from build123d import *

# Parameters (mm, degrees)
BOSS_EXTRUDE1_DEPTH = 279.4
SKETCH2_W           = 241.3
SKETCH2_H           = 124.206
SKETCH2_H_2         = 28.194
CUT_EXTRUDE3_DEPTH  = 80.368181
FILLET1_R           = 1.5875
SKETCH4_W           = 241.3
SKETCH4_H           = 84.002363795
CUT_EXTRUDE5_DEPTH  = 7.62


with BuildPart() as part:
    # Sketch1 → Boss-Extrude1 (new body)
    with BuildSketch(Plane(origin=(0, 0, 0), x_dir=(0, 0, -1), z_dir=(1, 0, 0))):
        with BuildLine():
            Line((0, 0), (101.6, 0))
            Line((101.6, 0), (152.4, 87.988181024))
            Line((152.4, 87.988181024), (124.206, 87.988181024))
            ThreePointArc((124.206, 87.988181024), (89.315487923, 46.885255226), (43.091610276, 74.636858378))
            Line((43.091610276, 74.636858378), (0, 0))
        make_face()
        with BuildLine():
            Line((139.201772846, 80.368181024), (131.23325971, 80.368181024))
            ThreePointArc((131.23325971, 80.368181024), (94.185048049, 40.105513671), (42.791899046, 58.8777433))
            Line((42.791899046, 58.8777433), (13.198227154, 7.62))
            Line((13.198227154, 7.62), (97.200590949, 7.62))
            Line((97.200590949, 7.62), (139.201772846, 80.368181024))
        make_face(mode=Mode.SUBTRACT)
    extrude(amount=BOSS_EXTRUDE1_DEPTH)

    # Sketch2 → Cut-Extrude3 (cut)
    with BuildSketch(Plane(origin=(0, 87.988181024, 0), x_dir=(1, 0, 0), z_dir=(0, 1, 0))):
        with Locations((139.7, 62.103)):
            Rectangle(SKETCH2_W, SKETCH2_H)
        with Locations((139.7, 138.303)):
            Rectangle(SKETCH2_W, SKETCH2_H_2)
    extrude(amount=-CUT_EXTRUDE3_DEPTH, mode=Mode.SUBTRACT)

    # Fillet1
    fillet1_edges = [part.edges().sort_by_distance(p)[0] for p in [
        (279.4, 46.885255226, -89.315487923),
        (9.525, 74.636858378, -43.091610276),
        (9.525, 87.988181024, -124.206),
        (19.05, 46.885255226, -89.315487923),
        (260.35, 46.885255226, -89.315487923),
        (0, 46.885255226, -89.315487923),
        (269.875, 74.636858378, -43.091610276),
        (269.875, 87.988181024, -124.206),
    ]]
    fillet(fillet1_edges, radius=FILLET1_R)

    # Sketch4 → Cut-Extrude5 (cut)
    with BuildSketch(Plane(origin=(0, 7.62, 0), x_dir=(1, 0, 0), z_dir=(0, 1, 0))):
        with Locations((139.7, 55.199409051)):
            Rectangle(SKETCH4_W, SKETCH4_H)
    extrude(amount=-CUT_EXTRUDE5_DEPTH, mode=Mode.SUBTRACT)


solid = part.part
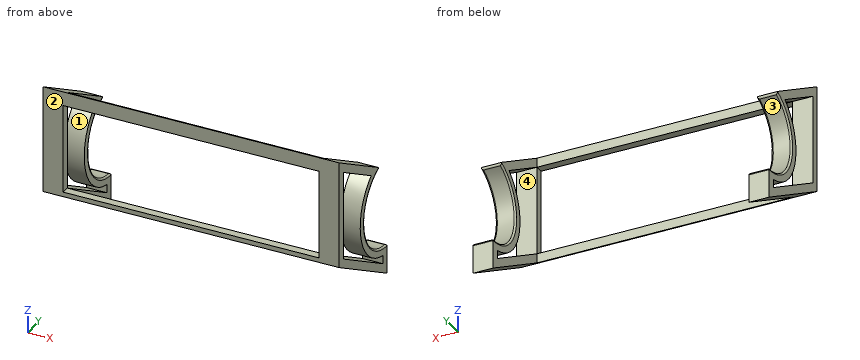
Design review of the part built by this model. Coordinates are the model's own, in mm. Face numbers are marked on the shaded views. A direction names the side the tool comes from. Coordinates: 2 decimals unless noted, no trailing zeros. Loops run counter-clockwise (first coordinate to the right, second up) from the corner with the lowest first, then second, coordinate; pieces in that order, holes last. Notation, with made-up numbers: (52, 33) -> (72, 33) arc R21 cw to (72, 56) -> close; hole circle Ø11 at (-11.5, 17.5). An arc over 180 degrees is marked (long way). Use a Markdown table: item, result. Add a question column.
Item 1: Clearance check with flat-ended pins moving along their axes: P1, Ø7, axis at x = 100.5, z = -100, coming from the +Y side; P2, Ø21, axis at x = 9, z = -44, coming from the +Y side; P3, Ø6, axis at x = 160, y = 4.5, coming from the +Z side. State where each tip first meets the part, or that it passes through.
Item 2: We need section C-C, the plane z = -34. Write out the cut boundary in (x, y), and give its area (3 significant figures).
Item 3: We need section D-D, the plane y = 20.5. Write out the cut boundary in (x, z).
Item 4: We need section B-B, the plane y = 42. Write out the cut boundary in (x, z), and give its area (3 significant figures).
Item 5: We need section A-A, the plane x = 34. Write out the cut boundary in (y, z), and give its area (3 significant figures).
Item 6: Machinability: for the marked faces 3 and 4, which of the approach directions +Z, -Z, +X, -X, +Y, -Y give a long, thin tool a straight path to every point of the face, cutting with its end or side? Answer none if there is none.
Item 7: The part is to be moulded in two halves that separate along Z. For the marked faces 1 and 2, say which applies: +Z half, -Z half, draft (parallel to the pull), parting line (faces both ways), or undercut.
Item 8: Wall thickness on L1, parallel to X at y = 4, z = -68; L2, parallel to Y at x = 123, z = -99.5; L3, parallel to Z at x = 76, y = 6: over which ranges is each line inside the solid? List them lowest first. Write a range as from..to.
Numbers:
| question | item | result |
|---|---|---|
| 1 | P1 | stops at y = 7.62 |
| 1 | P2 | stops at y = 72.55 |
| 1 | P3 | stops at z = -0.87 |
| 2 | outline | (0, 0) -> (19.05, 0) -> (19.05, 7.62) -> (0, 7.62) -> close; (0, 43.65) -> (19.05, 43.65) -> (19.05, 58.89) -> (0, 58.89) -> close; (260.35, 0) -> (279.4, 0) -> (279.4, 7.62) -> (260.35, 7.62) -> close; (260.35, 43.65) -> (279.4, 43.65) -> (279.4, 58.89) -> (260.35, 58.89) -> close |
| 2 | area | 871 mm^2 |
| 3 | outline | (0, -113.44) -> (19.05, -113.44) -> (19.05, -104.64) -> (0, -104.64) -> close; (0, -20.63) -> (19.05, -20.63) -> (19.05, -11.84) -> (0, -11.84) -> close; (260.35, -113.44) -> (279.4, -113.44) -> (279.4, -104.64) -> (260.35, -104.64) -> close; (260.35, -20.63) -> (279.4, -20.63) -> (279.4, -11.84) -> (260.35, -11.84) -> close |
| 4 | outline | (0, -125.85) -> (19.05, -125.85) -> (19.05, -117.05) -> (0, -117.05) -> close; (0, -100.25) -> (19.05, -100.25) -> (19.05, -64.85) -> (0, -64.85) -> close; (0, -33.05) -> (19.05, -33.05) -> (19.05, -24.25) -> (0, -24.25) -> close; (260.35, -125.85) -> (279.4, -125.85) -> (279.4, -117.05) -> (260.35, -117.05) -> close; (260.35, -100.25) -> (279.4, -100.25) -> (279.4, -64.85) -> (260.35, -64.85) -> close; (260.35, -33.05) -> (279.4, -33.05) -> (279.4, -24.25) -> (260.35, -24.25) -> close |
| 4 | area | 2,020 mm^2 |
| 5 | outline | (0, -101.6) -> (7.62, -106) -> (7.62, -97.2) -> (0, -97.2) -> close; (0, -13.2) -> (7.62, -13.2) -> (7.62, -4.4) -> (0, 0) -> close |
| 5 | area | 134 mm^2 |
| 6 | face 3 | +X, -X, +Y |
| 6 | face 4 | +X, -X |
| 7 | face 1 | undercut |
| 7 | face 2 | draft |
| 8 | L1 | x = 0..19.05, 260.35..279.4 |
| 8 | L2 | y = 0..7.62 |
| 8 | L3 | z = -105.06..-97.2, -13.2..-3.46 |
